Geometry check sheet. Reference: the model listing, model coordinates, mm. Face numbers are marked on the shaded views. A direction names the side the tool comes from. Round coordinates to 2 decimals unless told otherwise and drop trailing zeros. Order: outer loops, then holes, each group sorted by start corner. A loop starts at its lowest first (then second) coordinate and runs counter-clockwise, first axis right, second up. Notation, with made-up numbers: (11.5, 77.25) - (39.5, 77.25) arc R32 cw to (39.5, 107.25) - close; hole circle Ø9 at (13.5, -40). An arc over 180 degrees is marked (long way). Answer as CSV lines item,"result". Start each with the question number.
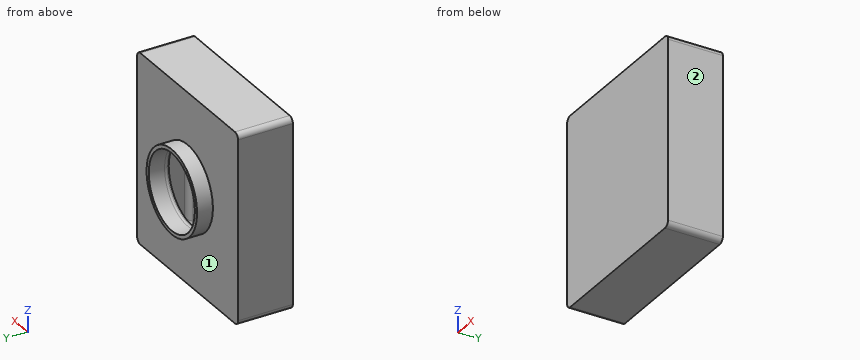
```python
from build123d import *

# Parameters (mm, degrees)
SKETCH1_W           = 203.2
SKETCH1_H           = 228.6
SKETCH1_W_2         = 190.5
SKETCH1_H_2         = 215.9
BOSS_EXTRUDE1_DEPTH = 53.34
SKETCH2_W           = 203.2
SKETCH2_H           = 228.6
BOSS_EXTRUDE2_DEPTH = 6.35
SKETCH3_W           = 203.2
SKETCH3_H           = 228.6
BOSS_EXTRUDE3_DEPTH = 6.35
CUT_EXTRUDE1_REACH  = 68.04
SKETCH5_R           = 46.355
FILLET5_R           = 6.35
SKETCH6_R           = 50.8
SKETCH6_R_2         = 46.355
BOSS_EXTRUDE4_DEPTH = 19.05
FILLET6_R           = 3.175


with BuildPart() as part:
    # Sketch1 → Boss-Extrude1 (new body)
    with BuildSketch(Plane(origin=(0, 0, 0), x_dir=(1, 0, 0), z_dir=(0, 1, 0))):
        with Locations((-54.462846348, 15.85288386)):
            Rectangle(SKETCH1_W, SKETCH1_H)
        with Locations((-54.462846348, 15.85288386)):
            Rectangle(SKETCH1_W_2, SKETCH1_H_2, mode=Mode.SUBTRACT)
    extrude(amount=BOSS_EXTRUDE1_DEPTH)

    # Sketch2 → Boss-Extrude2 (add)
    with BuildSketch(Plane(origin=(0, 0, 0), x_dir=(-1, 0, 0), z_dir=(0, -1, 0))):
        with Locations((54.462846348, 15.85288386)):
            Rectangle(SKETCH2_W, SKETCH2_H)
    extrude(amount=BOSS_EXTRUDE2_DEPTH)

    # Sketch3 → Boss-Extrude3 (add)
    with BuildSketch(Plane(origin=(0, 53.34, 0), x_dir=(1, 0, 0), z_dir=(0, 1, 0))):
        with Locations((-54.462846348, 15.85288386)):
            Rectangle(SKETCH3_W, SKETCH3_H)
    extrude(amount=BOSS_EXTRUDE3_DEPTH)

    # Sketch5 → Cut-Extrude1 (cut, up to next)
    with BuildSketch(Plane(origin=(0, 59.69, 0), x_dir=(1, 0, 0), z_dir=(0, 1, 0)), mode=Mode.PRIVATE) as cut_extrude1_sk1:
        with Locations((-54.462846348, 14.706120018)):
            Circle(SKETCH5_R)
    cut_extrude1_tool1 = extrude(cut_extrude1_sk1.sketch, amount=-CUT_EXTRUDE1_REACH, mode=Mode.PRIVATE) & part.part
    add(cut_extrude1_tool1.solids().sort_by_distance((-54.462846, 59.69, -14.70612))[0], mode=Mode.SUBTRACT)

    # Fillet5
    fillet5_edges = [part.edges().sort_by_distance(p)[0] for p in [
        (-149.712846348, 0, -15.85288386),
        (-149.712846348, 26.67, -123.80288386),
        (-54.462846348, 0, 92.09711614),
        (-149.712846348, 26.67, 92.09711614),
        (40.787153652, 0, -15.85288386),
        (40.787153652, 26.67, 92.09711614),
        (-54.462846348, 0, -123.80288386),
        (40.787153652, 26.67, -123.80288386),
        (-149.712846348, 53.34, -15.85288386),
        (-54.462846348, 53.34, 92.09711614),
        (40.787153652, 53.34, -15.85288386),
        (-54.462846348, 53.34, -123.80288386),
        (-156.062846348, 26.67, -130.15288386),
        (47.137153652, 26.67, -130.15288386),
        (47.137153652, 26.67, 98.44711614),
        (-156.062846348, 26.67, 98.44711614),
    ]]
    fillet(fillet5_edges, radius=FILLET5_R)

    # Sketch6 → Boss-Extrude4 (add)
    with BuildSketch(Plane(origin=(0, 59.69, 0), x_dir=(1, 0, 0), z_dir=(0, 1, 0))):
        with Locations((-54.462846348, 14.706120018)):
            Circle(SKETCH6_R)
        with Locations((-54.462846348, 14.706120018)):
            Circle(SKETCH6_R_2, mode=Mode.SUBTRACT)
    extrude(amount=BOSS_EXTRUDE4_DEPTH)

    # Fillet6
    fillet6_edges = [part.edges().sort_by_distance(p)[0] for p in [
        (-100.817846348, 53.34, -14.706120018),
    ]]
    fillet(fillet6_edges, radius=FILLET6_R)


solid = part.part
```
1. Section check A-A on z = 72. Record the boundary of the cut face in (x, y), plus the area to 3 significant figures.
2. Section check B-B on y = 10. Record the boundary of the cut face in (x, z).
3. Go/stop test with flat-tipped pins: pin 1 Ø6 at (x, z) = (-24.5, -104.5) entering from +Y; pin 2 Ø4 at (x, z) = (-32, -38.5) entering from +Y. Record where each tip stops, or that it passes through.
4. Access from +Z, -Z, +X, -X, +Y, -Y to the whole of each face (thin tool, end or side, straight path). Record for the marked faces 1 and 2.
5. Section check C-C on y = 68. Record the boundary of the cut face in (x, z) (3 decimals).
6. Thickness scan on probe 1 along X at (y, z) = (22, 22.5); probe 2 along Z at (x, y) = (27, 29.5); probe 3 along Y at (x, z) = (-113.5, 49.5). Record the ranges inside material, lowest first.
Numbers:
1,outline,"(-156.06, -6.35) - (47.14, -6.35) - (47.14, 59.69) - (-156.06, 59.69) - close; hole (-149.71, 6.35) arc R6.35 ccw to (-143.36, 0) - (34.44, 0) arc R6.35 ccw to (40.79, 6.35) - (40.79, 46.99) arc R6.35 ccw to (34.44, 53.34) - (-143.36, 53.34) arc R6.35 ccw to (-149.71, 46.99) - close"
1,area,"3,290 mm2"
2,outline,"(-156.06, -123.8) arc R6.35 ccw to (-149.71, -130.15) - (40.79, -130.15) arc R6.35 ccw to (47.14, -123.8) - (47.14, 92.1) arc R6.35 ccw to (40.79, 98.45) - (-149.71, 98.45) arc R6.35 ccw to (-156.06, 92.1) - close; hole (-149.71, -117.45) arc R6.35 ccw to (-143.36, -123.8) - (34.44, -123.8) arc R6.35 ccw to (40.79, -117.45) - (40.79, 85.75) arc R6.35 ccw to (34.44, 92.1) - (-143.36, 92.1) arc R6.35 ccw to (-149.71, 85.75) - close"
3,pin 1,"stops at y = 59.69"
3,pin 2,"stops at y = 0"
4,face 1,"+Y"
4,face 2,"+Z, -Z, +X, +Y, -Y"
5,outline,"circle Ø101.6 at (-54.463, -14.706); hole circle Ø92.71 at (-54.463, -14.706)"
6,probe 1,"x = -156.06 to -149.71, 40.79 to 47.14"
6,probe 2,"z = -130.15 to -123.8, 92.1 to 98.45"
6,probe 3,"y = -6.35 to 0, 53.34 to 59.69"
